from build123d import *

# Parameters (mm, degrees)
SCHIZZO2_R = 40
BASE_DEPTH = 29


with BuildPart() as part:
    # Schizzo2 → Base (new, symmetric)
    with BuildSketch(Plane.XY):
        with Locations(Location((0, 0, 0), (0, 0, 180))):
            Circle(SCHIZZO2_R)
    extrude(amount=BASE_DEPTH, both=True)

    # Schizzo3 → Rivoluzione1 (revolve)
    with BuildSketch(Plane.XY, mode=Mode.PRIVATE) as rivoluzione1_sk:
        with BuildLine():
            Line((40, 0), (51.818447633, 0))
            Line((51.818447633, 0), (51.818447633, -32.5))
            Line((51.818447633, -32.5), (23.318447633, -32.5))
            ThreePointArc((23.318447633, -32.5), (35.586078074, -18.265569998), (40, 0))
        make_face()
    revolve(rivoluzione1_sk.sketch.rotate(Axis((-78.446809676, 0, 0), (1, 0, 0)), 270), axis=Axis((-78.446809676, 0, 0), (1, 0, 0)))


solid = part.part
Read the model definition and answer for the solid it produces. Units are mm, in the model's axes. Give positions to 0.01 mm unless a question says otherwise; leave off trailing zeros. Loops run counter-clockwise (first coordinate to the right, second up) from the corner with the lowest first, then second, coordinate; pieces in that order, holes last. Notation, with made-up numbers: (-19, -6) - (-1, -6) arc R12 cw to (-1, 2) - close; hole circle Ø11 at (59, 71.25). An arc over 180 degrees is marked (long way). Answer as CSV lines item,"result". Start each with the question number.
1) Each of these flat-tipped pins is pushed along its axis until it touches: pin 1 Ø1.5 at (y, z) = (-4.5, -1) entering from -X; pin 2 Ø3 at (x, z) = (-29, 24) entering from +Y; pin 3 Ø4 at (y, z) = (4, 21) entering from -X; pin 4 Ø12 at (y, z) = (-27, -25.5) entering from +X. Where does it stop, or does it pass through?
2) Find section A-A (y = 0). Write down the section's boundary in (x, z).
3) Find section C-C (z = 0). Write down the section's boundary in (x, y), then the cut area to 3 significant figures.
4) Straight lines are drawn through the part: L1, parallel to Z at x = 20.5, y = -11; L2, parallel to X at y = 2, z = -3.5; L3, parallel to X at y = -35, z = -23. For each, find the intervals that lie inside material, in ascending order. Write a range as from..to.
5) Find section D-D (y = 29.5). Write down the section's boundary in (x, z).
6) Find section B-B (x = 0). Write down the section's boundary in (y, z), then the cut area to 3 significant figures.
7) Determine the mould class of faces 1 (the face through (51.818, 0, 0)), 2 (the face through (-39.97, 1.55, 0.41)) for opening direction X: released by +X, released by -X, zero draft, split by the parting line, or undercut.
Findings below:
1,pin 1,"x = -39.82"
1,pin 2,"y = 29.05"
1,pin 3,"x = -39.95"
1,pin 4,"x = 51.82"
2,outline,"(-40, -29) - (27.55, -29) arc R40 cw to (23.32, -32.5) - (51.82, -32.5) - (51.82, 32.5) - (23.32, 32.5) arc R40 cw to (27.55, 29) - (-40, 29) - close"
3,outline,"(23.32, -32.5) - (51.82, -32.5) - (51.82, 32.5) - (23.32, 32.5) arc R40 ccw (long way) to start"
3,area,"6,120 mm^2"
4,L1,"-29..29"
4,L2,"-39.95..51.82"
4,L3,"-19.36..19.36"
5,outline,"(-27.01, -29) - (27.01, -29) - (27.01, -13.64) - (51.82, -13.64) - (51.82, 13.64) - (27.01, 13.64) - (27.01, 29) - (-27.01, 29) - close"
6,outline,"(-40, -29) - (40, -29) - (40, 29) - (-40, 29) - close"
6,area,"4,640 mm^2"
7,face 1,"released by +X"
7,face 2,"split by the parting line"
